from build123d import *

# Parameters (mm, degrees)
F0_W     = 610
F0_H     = 210
F1_DEPTH = 10
F2_W     = 10
F2_H     = 105
F3_DEPTH = 25
F5_D     = 2
F5_DEPTH = 12
F5_TIP   = 0.600860619
F7_D     = 2
F7_DEPTH = 12
F7_TIP   = 0.600860619


with BuildPart() as f1:
    # F0 (on Front) → F1 (new body)
    with BuildSketch(Plane.XZ):
        with Locations((-305, 105)):
            Rectangle(F0_W, F0_H)
    extrude(amount=F1_DEPTH)

    # F2 (on face) → F3 (cut)
    with BuildSketch(Plane.XZ.offset(10)):
        with Locations((-530, 52.5)):
            Rectangle(F2_W, F2_H)
        with Locations((-455, 52.5)):
            Rectangle(F2_W, F2_H)
        with Locations((-380, 52.5)):
            Rectangle(F2_W, F2_H)
        with Locations((-230, 52.5)):
            Rectangle(F2_W, F2_H)
        with Locations((-155, 52.5)):
            Rectangle(F2_W, F2_H)
        with Locations((-305, 52.5)):
            Rectangle(F2_W, F2_H)
        with Locations((-80, 52.5)):
            Rectangle(F2_W, F2_H)
    extrude(amount=-F3_DEPTH, mode=Mode.SUBTRACT)

    # F5
    with Locations(Plane(origin=(-610, 0, 0), x_dir=(0, -1, 0), z_dir=(-1, 0, 0))):
        with Locations((5, 190), (5, 20)):
            Hole(F5_D / 2, depth=F5_DEPTH)
            with Locations((0, 0, -(F5_DEPTH + F5_TIP / 2))):  # 118° drill point
                Cone(0, F5_D / 2, F5_TIP, mode=Mode.SUBTRACT)

    # F7
    with Locations(Plane.YZ):
        with Locations((-5, 190), (-5, 20)):
            Hole(F7_D / 2, depth=F7_DEPTH)
            with Locations((0, 0, -(F7_DEPTH + F7_TIP / 2))):  # 118° drill point
                Cone(0, F7_D / 2, F7_TIP, mode=Mode.SUBTRACT)


solid = f1.part
Read the model definition and answer for the solid it produces. Units are mm, in the model's axes. A direction names the side the tool comes from. Give positions to 0.01 mm unless a question says otherwise; leave off trailing zeros. Use CSV: the item, a comma, the result in double quotes. Start each with the question number.
Item 1: The part is cut by section A-A, the plane z = 83.5. Count the separate pieces of the cut face and the enclosed holes in it, and give its area (3 significant figures).
Item 2: Flat-ended cylindrical pins translate along their axes: P1, Ø5, axis at x = -380.5, y = -3.5, coming from the -Z side; P2, Ø1.8, axis at y = -5, z = 190, coming from the +X side. Find the tip coordinate at first contact, or state that the pin passes through.
Item 3: Consider line 1 (Z direction, x = -606.5, y = -5); line 2 (Y direction, x = -600, z = 20); line 3 (Z direction, x = -451.5, y = -0.5). Determine where each line is inside the solid, lowest interval first.
Item 4: The mould has two halves that part along X. Classify faces 1 (the flat face through (-80, -5, 105)), 2 (the flat face through (-573, -5, 0)): pulls with the +X half, pulls with the -X half, needs draft (parallel to the pull), parting line crosses it, or undercut.
Item 5: For faces 3 (the flat face through (-309, 0, 106)), 4 (the flat face through (-155, -5, 105)), determine the directions among +Z, -Z, +X, -X, +Y, -Y from which every point of the face is accessible in a straight line to the end or side of a thin tool.
Taken from the geometry:
1,separate pieces,"8"
1,enclosed holes,"0"
1,area,"5,400 mm2"
2,P1,"z = 105"
2,P2,"x = -12.06"
3,line 1,"0 to 19, 21 to 189, 191 to 210"
3,line 2,"-10 to -6, -4 to 0"
3,line 3,"105 to 210"
4,face 1,"undercut"
4,face 2,"needs draft"
5,face 3,"+Z, -Z, +X, -X, +Y"
5,face 4,"-Z, +Y, -Y"
